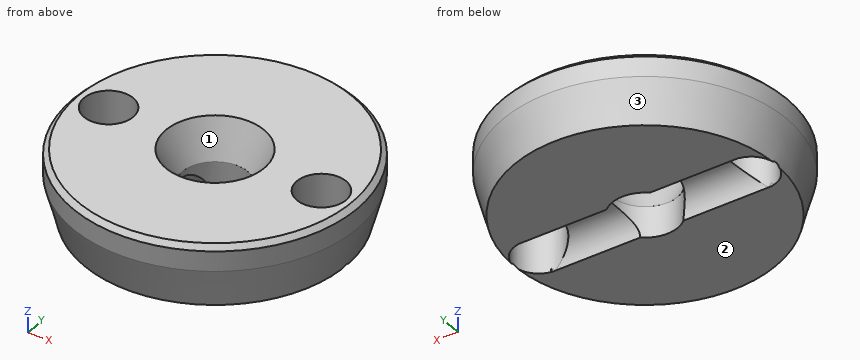
from build123d import *

# Parameters (mm, degrees)
F2_SIZE  = 0.3
F3_R     = 1.5
F4_DEPTH = 80
F5_R     = 1.5
F6_DEPTH = 6.75


with BuildPart() as f1:
    # F0 (on Front) → F1 (revolve)
    with BuildSketch(Plane.XZ):
        Polygon((-3, 53), (-7.65, 53), (-8.65, 53), (-8.65, 51.483571), (-7.975725, 48.967142), (-2, 48.967142), (-2, 50.855493), align=None)
    revolve(axis=Axis((0, 0, 14.86109), (0, 0, -1)))

    # F2
    f2_edges = [f1.edges().sort_by_distance(p)[0] for p in [
        (8.65, 0, 53),
    ]]
    chamfer(f2_edges, length=F2_SIZE)

    # F3 (on Top) → F4 (cut)
    with BuildSketch(Plane.XY):
        with Locations((-6.5, 0)):
            Circle(F3_R)
        with BuildLine():
            ThreePointArc((8, 0), (6.5, 1.5), (5, 0))
            ThreePointArc((5, 0), (6.5, -1.5), (8, 0))
        make_face()
    extrude(amount=F4_DEPTH, mode=Mode.SUBTRACT)

    # F5 (on Right) → F6 (cut, symmetric)
    with BuildSketch(Plane.YZ):
        with Locations((0, 48.971336)):
            Circle(F5_R)
    extrude(amount=F6_DEPTH, both=True, mode=Mode.SUBTRACT)


solid = f1.part
Verification items for the finished model (mm, model axes). Face numbers are marked on the shaded views. Give positions to 0.01 mm unless a question says otherwise; leave off trailing zeros. Write each loop counter-clockwise with the first axis right and the second up, starting at its lowest first coordinate (ties: lowest second). Pieces come first, ordered by that corner, then holes. Notation, with made-up numbers: (42.25, 68.25) - (73.25, 68.25) arc R28 ccw to (73.25, 93.25) - close; hole circle Ø2 at (-10.75, -11.75). An arc over 180 degrees is marked (long way). Answer as CSV lines item,"result". Start each with the question number.
1. Thickness scan on line 1 (Y direction, x = -7.5, z = 51.6); line 2 (Y direction, x = -6.5, z = 50.5); line 3 (X direction, y = -3, z = 51.85). Record the ranges inside material, lowest first.
2. Sectioned sample at A-A (x = 0). Record the boundary of the cut face in (y, z).
3. Depth check by flat-ended pin: pin 1 (2.5 mm diameter, centred on x = -6.5, y = 0, fed in from +Z); pin 2 (1 mm diameter, centred on x = -1, z = 51.5, fed in from -Y); pin 3 (1.5 mm diameter, centred on y = -2.5, z = 49.5, fed in from -X); pin 4 (1.5 mm diameter, centred on x = -3, z = 50.5, fed in from +Y). Enter the tip coordinate at first touch or a pass-through.
4. Draft check along X on the marked faces 1, 2 and 3. Enter one of: pulls with the +X half, pulls with the -X half, needs draft (parallel to the pull), parting line crosses it, or undercut.
5. Sectioned sample at B-B (y = 0). Record the boundary of the cut face in (x, z), then the cut area to 3 significant figures.
Derived:
1,line 1,"-4.31 to -1.12, 1.12 to 4.31"
1,line 2,"-5.3 to -1.5, 1.5 to 5.3"
1,line 3,"-8.11 to 8.11"
2,outline,"(-8.65, 51.48) - (-7.98, 48.97) - (-2, 48.97) - (-2, 50.86) - (-3, 53) - (-8.35, 53) - (-8.65, 52.7) - close; (2, 48.97) - (7.98, 48.97) - (8.65, 51.48) - (8.65, 52.7) - (8.35, 53) - (3, 53) - (2, 50.86) - close"
3,pin 1,"through"
3,pin 2,"y = -8.64"
3,pin 3,"x = -8.02"
3,pin 4,"y = 8.16"
4,face 1,"undercut"
4,face 2,"needs draft"
4,face 3,"parting line crosses it"
5,outline,"(-8.65, 51.48) - (-8, 49.06) - (-8, 53) - (-8.35, 53) - (-8.65, 52.7) - close; (-5, 50.47) - (-2, 50.47) - (-2, 50.86) - (-3, 53) - (-5, 53) - close; (2, 50.47) - (5, 50.47) - (5, 53) - (3, 53) - (2, 50.86) - close; (8, 49.06) - (8.65, 51.48) - (8.65, 52.7) - (8.35, 53) - (8, 53) - close"
5,area,"16.5 mm²"
